```python
from build123d import *

# Parameters (mm, degrees)
EL_MENT_M_CANO_SOUD_1_DEPTH     = 200
ESQUISSE2_W                     = 60
ESQUISSE2_H                     = 10
ENL_V_MAT_EXTRU_1_DEPTH         = 60
DIAM_TRE_DU_PER_AGE_14_0_14_1_D = 14


with BuildPart() as part:
    # Sketch1 → Elément mécano-soudé1 (new body)
    with BuildSketch(Plane.YZ.offset(-100)):
        with BuildLine():
            Line((-20, -30), (20, -30))
            ThreePointArc((20, -30), (27.071067812, -27.071067812), (30, -20))
            Line((30, -20), (30, 20))
            ThreePointArc((30, 20), (27.071067812, 27.071067812), (20, 30))
            Line((20, 30), (-20, 30))
            ThreePointArc((-20, 30), (-27.071067812, 27.071067812), (-30, 20))
            Line((-30, 20), (-30, -20))
            ThreePointArc((-30, -20), (-27.071067812, -27.071067812), (-20, -30))
        make_face()
        with BuildLine():
            Line((-20, -25), (20, -25))
            ThreePointArc((20, -25), (23.535533906, -23.535533906), (25, -20))
            Line((25, -20), (25, 20))
            ThreePointArc((25, 20), (23.535533906, 23.535533906), (20, 25))
            Line((20, 25), (-20, 25))
            ThreePointArc((-20, 25), (-23.535533906, 23.535533906), (-25, 20))
            Line((-25, 20), (-25, -20))
            ThreePointArc((-25, -20), (-23.535533906, -23.535533906), (-20, -25))
        make_face(mode=Mode.SUBTRACT)
    extrude(amount=EL_MENT_M_CANO_SOUD_1_DEPTH)

    # Esquisse2 → Enlèv. mat.-Extru.1 (cut)
    with BuildSketch(Plane(origin=(-100, 0, 0), x_dir=(0, 0, -1), z_dir=(1, 0, 0))):
        with Locations((0, -25)):
            Rectangle(ESQUISSE2_W, ESQUISSE2_H)
    enl_v_mat_extru_1 = extrude(amount=ENL_V_MAT_EXTRU_1_DEPTH, mode=Mode.SUBTRACT)

    # Diamètre du perçage Ø14.0 (14)1 (through all)
    with Locations(Plane.XY.offset(30)):
        with Locations((-80, 0), (80, 0)):
            Hole(DIAM_TRE_DU_PER_AGE_14_0_14_1_D / 2)

    # Symétrie1: Enlèv. mat.-Extru.1 across plane
    add(enl_v_mat_extru_1.mirror(Plane(origin=(0, 0, 0), x_dir=(0, 0, 1), z_dir=(1, 0, 0))), mode=Mode.SUBTRACT)


solid = part.part
```
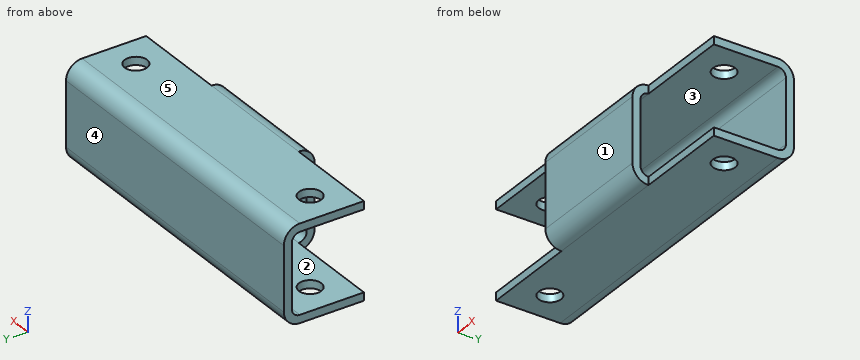
Verification items for the finished model (mm, model axes). Face numbers are marked on the shaded views. A direction names the side the tool comes from. Round coordinates to 2 decimals unless told otherwise and drop trailing zeros. Order: outer loops, then holes, each group sorted by start corner. A loop starts at its lowest first (then second) coordinate and runs counter-clockwise, first axis right, second up.
1) Cross-section at A-A, the plane y = -11. Record the cut outline in (x, z).
Geometry says:
outline: (-100, -30) - (100, -30) - (100, -25) - (-100, -25) - close; (-100, 25) - (100, 25) - (100, 30) - (-100, 30) - close
2) Draft check along Y on the marked faces 3, 4 and 5. Enter one of: +Y half, -Y half, draft (parallel to the pull), parting line (faces both ways), or undercut.
Geometry says:
face 3: undercut
face 4: +Y half
face 5: draft
3) Depth check by flat-ended pin: pin 1 (3 mm diameter, centred on y = -27, z = 10, fed in from -X); pin 2 (1 mm diameter, centred on x = -6, y = 22, fed in from +Z); pin 3 (1.5 mm diameter, centred on x = -63.5, z = 26.5, fed in from -Y); pin 4 (12.5 mm diameter, centred on x = -80, y = 0, fed in from -Z). Enter the tip coordinate at first touch or a pass-through.
Geometry says:
pin 1: stops at x = -40
pin 2: stops at z = 29.89
pin 3: stops at y = -20
pin 4: passes through
4) Cross-section at B-B, the plane x = 14. Record the cut outline in (y, z), plus the area to 3 significant figures.
Geometry says:
outline: (-30, -20) arc R10 ccw to (-20, -30) - (20, -30) arc R10 ccw to (30, -20) - (30, 20) arc R10 ccw to (20, 30) - (-20, 30) arc R10 ccw to (-30, 20) - close; hole (-25, -20) arc R5 ccw to (-20, -25) - (20, -25) arc R5 ccw to (25, -20) - (25, 20) arc R5 ccw to (20, 25) - (-20, 25) arc R5 ccw to (-25, 20) - close
area: 1,040 mm2
5) Cross-section at D-D, the plane y = 0. Record the cut outline in (x, z).
Geometry says:
outline: (-100, -30) - (-87, -30) - (-87, -25) - (-100, -25) - close; (-100, 25) - (-87, 25) - (-87, 30) - (-100, 30) - close; (-73, -30) - (73, -30) - (73, -25) - (-73, -25) - close; (-73, 25) - (73, 25) - (73, 30) - (-73, 30) - close; (87, -30) - (100, -30) - (100, -25) - (87, -25) - close; (87, 25) - (100, 25) - (100, 30) - (87, 30) - close
6) Tool access check on the marked faces 1 and 2. Record the directions out of +Z, -Z, +X, -X, +Y, -Y that give a thin tool (end or side, any length) a straight path to the whole face; none if there is none.
Geometry says:
face 1: +Z, -Z, +X, -X, -Y
face 2: +X, -X
7) Cross-section at C-C, the plane z = -9. Record the cut outline in (x, y), plus the area to 3 significant figures.
Geometry says:
outline: (-100, 25) - (100, 25) - (100, 30) - (-100, 30) - close; (-40, -30) - (40, -30) - (40, -25) - (-40, -25) - close
area: 1,400 mm2
8) Material ranges on line 1 (Z direction, x = -49.5, y = 18); line 2 (Y direction, x = -52, z = 1.5), recorded low to high.
Geometry says:
line 1: z = -30 to -25, 25 to 30
line 2: y = 25 to 30
